```python
from build123d import *

# Parameters (mm, degrees)
SKETCH1_W               = 200
SKETCH1_H               = 100
BOSS_EXTRUDE1_DEPTH     = 2.6
FILLET1_R               = 10
SKETCH6_R               = 1.5
CUT_EXTRUDE6_DEPTH      = 2.6
MIRROR6_COPY_1_SKETCH_R = 1.5
MIRROR6_COPY_1_DEPTH    = 2.6
SKETCH16_R              = 1.61925
CUT_EXTRUDE9_DEPTH      = 10
SKETCH17_R              = 1.61925
CUT_EXTRUDE10_DEPTH     = 224.621913059
SKETCH18_R              = 1.61925
CUT_EXTRUDE11_DEPTH     = 224.621913059
SKETCH19_R              = 1.61925
CUT_EXTRUDE12_DEPTH     = 224.621913059
SKETCH15_R              = 10
CUT_EXTRUDE14_DEPTH     = 224.621913059
SKETCH23_R              = 1.524
CUT_EXTRUDE15_DEPTH     = 2.59999988
MIRROR8_COPY_1_SKETCH_R = 1.524
MIRROR8_COPY_1_DEPTH    = 2.59999988


with BuildPart() as part:
    # Sketch1 → Boss-Extrude1 (new body)
    with BuildSketch(Plane(origin=(0, 0, 0), x_dir=(1, 0, 0), z_dir=(0, 1, 0))):
        with Locations((100, -50)):
            Rectangle(SKETCH1_W, SKETCH1_H)
    extrude(amount=BOSS_EXTRUDE1_DEPTH)

    # Fillet1
    fillet1_edges = [part.edges().sort_by_distance(p)[0] for p in [
        (0, 1.3, 0),
        (200, 1.3, 0),
        (200, 1.3, 100),
        (0, 1.3, 100),
    ]]
    fillet(fillet1_edges, radius=FILLET1_R)

    # Sketch6 → Cut-Extrude6 (cut)
    with BuildSketch(Plane.XZ):
        with Locations(Location((190, 10, 0), (0, 0, 270))):
            Circle(SKETCH6_R)
    cut_extrude6 = extrude(amount=-CUT_EXTRUDE6_DEPTH, mode=Mode.SUBTRACT)

    # Mirror5: Cut-Extrude6 across plane
    add(cut_extrude6.mirror(Plane(origin=(100, 0, 0), x_dir=(0, 0, 1), z_dir=(1, 0, 0))), mode=Mode.SUBTRACT)

    # Mirror6: Cut-Extrude6 across plane
    add(cut_extrude6.mirror(Plane.XY.offset(50)), mode=Mode.SUBTRACT)

    # Mirror6 copy 1 sketch → Mirror6 copy 1 (cut)
    with BuildSketch(Plane(origin=(200, 0, 100), x_dir=(-1, 0, 0), z_dir=(0, -1, 0))):
        with Locations(Location((190, 10, 0), (0, 0, 270))):
            Circle(MIRROR6_COPY_1_SKETCH_R)
    extrude(amount=-MIRROR6_COPY_1_DEPTH, mode=Mode.SUBTRACT)

    # Sketch16 → Cut-Extrude9 (cut)
    with BuildSketch(Plane(origin=(0, 2.6, 0), x_dir=(1, 0, 0), z_dir=(0, 1, 0))):
        with Locations(Location((35.15745, -29.37145, 0), (0, 0, 270))):
            Circle(SKETCH16_R)
    extrude(amount=-CUT_EXTRUDE9_DEPTH, mode=Mode.SUBTRACT)

    # Sketch17 → Cut-Extrude10 (cut, through all)
    with BuildSketch(Plane(origin=(0, 2.6, 0), x_dir=(1, 0, 0), z_dir=(0, 1, 0))):
        with Locations(Location((85.94475, -44.61145, 0), (0, 0, 270))):
            Circle(SKETCH17_R)
    extrude(amount=-CUT_EXTRUDE10_DEPTH, mode=Mode.SUBTRACT)

    # Sketch18 → Cut-Extrude11 (cut, through all)
    with BuildSketch(Plane(origin=(0, 2.6, 0), x_dir=(1, 0, 0), z_dir=(0, 1, 0))):
        with Locations(Location((34.01445, -77.28855, 0), (0, 0, 270))):
            Circle(SKETCH18_R)
    extrude(amount=-CUT_EXTRUDE11_DEPTH, mode=Mode.SUBTRACT)

    # Sketch19 → Cut-Extrude12 (cut, through all)
    with BuildSketch(Plane(origin=(0, 2.6, 0), x_dir=(1, 0, 0), z_dir=(0, 1, 0))):
        with Locations(Location((85.94475, -72.53875, 0), (0, 0, 270))):
            Circle(SKETCH19_R)
    extrude(amount=-CUT_EXTRUDE12_DEPTH, mode=Mode.SUBTRACT)

    # Sketch15 → Cut-Extrude14 (cut, through all)
    with BuildSketch(Plane.XZ):
        with Locations(Location((100, 50, 0), (0, 0, 270))):
            Circle(SKETCH15_R)
    extrude(amount=-CUT_EXTRUDE14_DEPTH, mode=Mode.SUBTRACT)

    # Sketch23 → Cut-Extrude15 (cut)
    with BuildSketch(Plane(origin=(0, 2.6, 0), x_dir=(1, 0, 0), z_dir=(0, 1, 0))):
        with Locations(Location((18.288, -9.906, 0), (0, 0, 270))):
            Circle(SKETCH23_R)
    cut_extrude15 = extrude(amount=-CUT_EXTRUDE15_DEPTH, mode=Mode.SUBTRACT)

    # Mirror7: Cut-Extrude15 across plane
    add(cut_extrude15.mirror(Plane(origin=(100, 0, 0), x_dir=(0, 0, 1), z_dir=(1, 0, 0))), mode=Mode.SUBTRACT)

    # Mirror8: Cut-Extrude15 across plane
    add(cut_extrude15.mirror(Plane.XY.offset(50)), mode=Mode.SUBTRACT)

    # Mirror8 copy 1 sketch → Mirror8 copy 1 (cut)
    with BuildSketch(Plane(origin=(200, 2.6, 100), x_dir=(-1, 0, 0), z_dir=(0, 1, 0))):
        with Locations(Location((18.288, -9.906, 0), (0, 0, 270))):
            Circle(MIRROR8_COPY_1_SKETCH_R)
    extrude(amount=-MIRROR8_COPY_1_DEPTH, mode=Mode.SUBTRACT)


solid = part.part
```
Build history of the part. All positions in model axes, mm. Round coordinates to 2 decimals unless told otherwise and drop trailing zeros. Write each loop counter-clockwise with the first axis right and the second up, starting at its lowest first coordinate (ties: lowest second). Pieces come first, ordered by that corner, then holes. Notation, with made-up numbers: (17, 22.5) - (58, 22.5) arc R22 ccw to (58, 46.5) - close; hole circle Ø3 at (70.5, 17). An arc over 180 degrees is marked (long way). Answer as CSV lines item,"result".
Q1. Cut at B-B (x = 100). Write the cut outline in (y, z), and give its area (3 significant figures).
Report:
outline,"(0, 0) - (2.6, 0) - (2.6, 40) - (0, 40) - close; (0, 60) - (2.6, 60) - (2.6, 100) - (0, 100) - close"
area,"208 mm^2"
Q2. Drop a flat-ended pin along its axis: pin 1 (12 mm diameter, centred on x = 100, z = 50, fed in from +Y). Give the stop position or say it passes through.
Report:
pin 1,"passes through"
Q3. Cut at A-A (z = 50). Write the cut outline in (x, y), and give its area (3 significant figures).
Report:
outline,"(0, 0) - (90, 0) - (90, 2.6) - (0, 2.6) - close; (110, 0) - (200, 0) - (200, 2.6) - (110, 2.6) - close"
area,"468 mm^2"
Q4. Pull direction X, two halves, no side cores. Call faces 1 (the cylindrical face through (197.15, 1.32, 3.01)), 2 (the flat face through (99, 2.6, 38)), 3 (the cylindrical face through (109.915, 1.282, 51.302)), 4 (the cylindrical face through (2.85, 1.32, 3.01)): +X half, -X half, draft (parallel to the pull), parting line (faces both ways), or undercut.
Report:
face 1,"+X half"
face 2,"draft"
face 3,"undercut"
face 4,"-X half"
Q5. Drill centre lines: probe 1 along X at (y, z) = (0.8, 10); probe 2 along Z at (x, y) = (190, 1.7); probe 3 along X at (y, z) = (0.85, 91). Where is each one in solid material? Low to high. Write a range as [from, to].
Report:
probe 1,"x = [0, 8.5], [11.5, 16.77], [19.81, 180.19], [183.23, 188.5], [191.5, 200]"
probe 2,"z = [0, 8.5], [11.5, 88.5], [91.5, 100]"
probe 3,"x = [0.05, 8.88], [11.12, 17.06], [19.51, 180.49], [182.94, 188.88], [191.12, 199.95]"
Q6. Cut at C-C (y = 2.15). State how many separate pieces and enclosed holes the cut face has, and give its area (3 significant figures).
Report:
separate pieces,"1"
enclosed holes,"13"
area,"19,500 mm^2"
